Can you work these out from the drawing? Everything is in mm from the part's minimum corner. A direction names the side the tool comes from. Coordinates: 2 decimals unless noted, no trailing zeros. Order: outer loops, then holes, each group sorted by start corner. A loop starts at its lowest first (then second) coordinate and runs counter-clockwise, first axis right, second up. Notation, with made-up numbers: (86.5, 62) -> (115.5, 62) arc R16 cw to (115.5, 87) -> close; hole circle Ø7 at (16, 15). An arc over 180 degrees is marked (long way). Use a Markdown table: item, result. Add a question column.
1) Thinking about a two-plate mould opening in X: for the marked faces 4, 5 and 6, which applies, +X half, -X half, draft (parallel to the pull), parting line (faces both ways), or undercut?
2) If we section it at C-C (z = 10.75): Write out the boundary of the cut face in (x, y), plus the area to 3 significant figures.
3) Will these pins go through, and if not, where does the flat tip stop? pin 1 Ø2 at (y, z) = (10, 20.5) entering from -X; pin 2 Ø1 at (x, y) = (3, 13.5) entering from +Z; pin 3 Ø3 at (y, z) = (5, 13.5) entering from -X.
4) Which directions (+Z, -Z, +X, -X, +Y, -Y) give clear straight access to the entire face, cutting with the end or side of a thin tool? Please do the marked faces 1, 2 and 3.
5) If I drill on L1, parallel to Y at x = 12.5, z = 6.5; L2, parallel to X at y = 12.5, z = 13.25, over which ranges is the centre line in solid material (lowest first)? Write a range as [from, to].
6) If we section it at D-D (z = 2.5): Write out the boundary of the cut face in (x, y), plus the area to 3 significant figures.
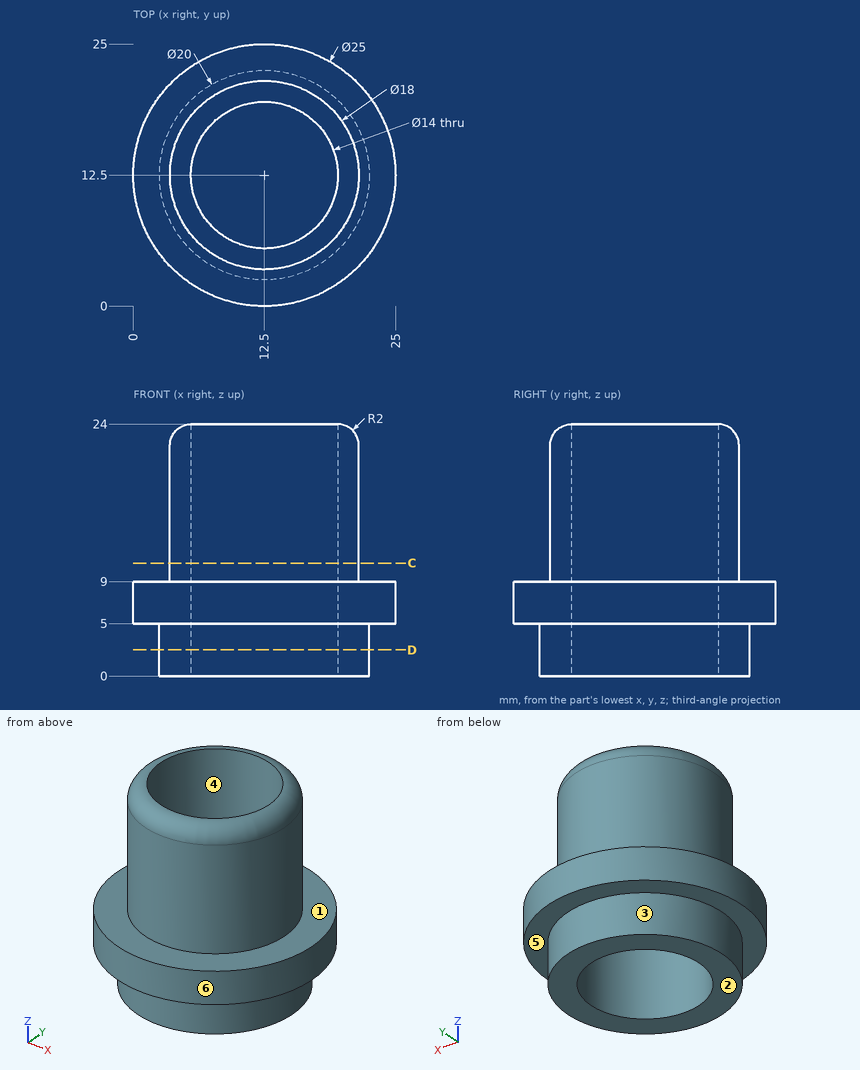
Answer sheet:
| question | item | result |
|---|---|---|
| 1 | face 4 | undercut |
| 1 | face 5 | draft |
| 1 | face 6 | parting line |
| 2 | outline | circle Ø18 at (12.5, 12.5); hole circle Ø14 at (12.5, 12.5) |
| 2 | area | 101 mm2 |
| 3 | pin 1 | x = 3.63 |
| 3 | pin 2 | z = 9 |
| 3 | pin 3 | x = 5.79 |
| 4 | face 1 | +Z |
| 4 | face 2 | -Z, +X, -X, +Y, -Y |
| 4 | face 3 | -Z |
| 5 | L1 | [0, 5.5], [19.5, 25] |
| 5 | L2 | [3.5, 5.5], [19.5, 21.5] |
| 6 | outline | circle Ø20 at (12.5, 12.5); hole circle Ø14 at (12.5, 12.5) |
| 6 | area | 160 mm2 |
